Source: CAD feature listing. Evaluate the final solid. Frame: model axes, mm. A direction names the side the tool comes from. Coordinates: 2 decimals unless noted, no trailing zeros. Loops run counter-clockwise (first coordinate to the right, second up) from the corner with the lowest first, then second, coordinate; pieces in that order, holes last.
from build123d import *

# Parameters (mm, degrees)
SKETCH1_W             = 64.8
SKETCH1_H             = 12.6
BOSS_EXTRUDE1_DEPTH   = 2
SKETCH2_W             = 64.8
SKETCH2_H             = 12.6
SKETCH2_W_2           = 60.8
SKETCH2_H_2           = 8.6
BOSS_EXTRUDE2_DEPTH   = 8
CUT_EXTRUDE1_DEPTH    = 67.766758196
BOSS_EXTRUDE3_DEPTH   = 5
BOSS_EXTRUDE3_DRAFT   = 5
BOSS_EXTRUDE3_2_DEPTH = 5
BOSS_EXTRUDE3_2_DRAFT = 5
SKETCH5_R             = 1
CUT_EXTRUDE2_DEPTH    = 4
SKETCH6_W             = 8.6
SKETCH6_H             = 4
CUT_EXTRUDE3_DEPTH    = 3


# Read off the part's stored shape, not the designer's step: Boss-Extrude3
with BuildPart() as part:
    # Sketch1 → Boss-Extrude1 (new body)
    with BuildSketch(Plane(origin=(0, 0, 0), x_dir=(1, 0, 0), z_dir=(0, 1, 0))):
        with Locations((32.4, -6.3)):
            Rectangle(SKETCH1_W, SKETCH1_H)
    extrude(amount=BOSS_EXTRUDE1_DEPTH)

    # Sketch2 → Boss-Extrude2 (add)
    with BuildSketch(Plane(origin=(0, 2, 0), x_dir=(1, 0, 0), z_dir=(0, 1, 0))):
        with Locations((32.4, -6.3)):
            Rectangle(SKETCH2_W, SKETCH2_H)
        with Locations((32.4, -6.3)):
            Rectangle(SKETCH2_W_2, SKETCH2_H_2, mode=Mode.SUBTRACT)
    extrude(amount=BOSS_EXTRUDE2_DEPTH)

    # Sketch3 → Cut-Extrude1 (cut, through all)
    with BuildSketch(Plane(origin=(0, 0, 0), x_dir=(-1, 0, 0), z_dir=(0, -1, 0))):
        with BuildLine():
            ThreePointArc((-24.41, -6.4), (-24.964257247, -4.052128624), (-26.51, -2.2))
            Line((-26.51, -2.2), (-32.81, -2.2))
            ThreePointArc((-32.81, -2.2), (-34.907554575, -6.239778319), (-33.060367627, -10.4))
            Line((-33.060367627, -10.4), (-26.259632373, -10.4))
            ThreePointArc((-26.259632373, -10.4), (-24.894791188, -8.60347112), (-24.41, -6.4))
        make_face()
        with BuildLine():
            ThreePointArc((-33.060367627, -10.4), (-29.66, -11.65), (-26.259632373, -10.4))
            Line((-26.259632373, -10.4), (-33.060367627, -10.4))
        make_face()
        with BuildLine():
            Line((-32.81, -2.2), (-26.51, -2.2))
            ThreePointArc((-26.51, -2.2), (-29.66, -1.15), (-32.81, -2.2))
        make_face()
    extrude(amount=-CUT_EXTRUDE1_DEPTH, mode=Mode.SUBTRACT)


with BuildPart() as boss_extrude3_tool:
    # Boss-Extrude3 outline → Boss-Extrude3 (with draft: the straight prism first)
    with BuildSketch(Plane(origin=(0, 7, 0), x_dir=(1, 0, 0), z_dir=(0, 1, 0))):
        with BuildLine():
            Line((58.936583966, -10.162556682), (61.663416034, -10.162556682))
            ThreePointArc((61.663416034, -10.162556682), (62.076528267, -9.738845855), (62.362556682, -9.220791486))
            Line((62.362556682, -9.220791486), (62.362556682, -7.619208514))
            ThreePointArc((62.362556682, -7.619208514), (61.800640796, -6.794120462), (60.933251192, -6.3))
            ThreePointArc((60.933251192, -6.3), (61.800640796, -5.805879538), (62.362556682, -4.980791486))
            Line((62.362556682, -4.980791486), (62.362556682, -3.379208514))
            ThreePointArc((62.362556682, -3.379208514), (62.076528267, -2.861154145), (61.663416034, -2.437443318))
            Line((61.663416034, -2.437443318), (58.936583966, -2.437443318))
            ThreePointArc((58.936583966, -2.437443318), (58.125947095, -4.590975715), (59.666748808, -6.3))
            ThreePointArc((59.666748808, -6.3), (58.125947095, -8.009024285), (58.936583966, -10.162556682))
        make_face()
    extrude(amount=-BOSS_EXTRUDE3_DEPTH)
    # Boss-Extrude3: the draft: its side faces are tilted about the plane it starts from
    boss_extrude3_sides = [boss_extrude3_tool.faces().sort_by_distance(p)[0] for p in [
        (60.3, 4.5, 10.162556682),
        (62.076528267, 4.5, 9.738845855),
        (62.362556682, 4.5, 8.42),
        (61.800640796, 4.5, 6.794120462),
        (61.800640796, 4.5, 5.805879538),
        (62.362556682, 4.5, 4.18),
        (62.076528267, 4.5, 2.861154145),
        (60.3, 4.5, 2.437443318),
        (58.125947095, 4.5, 4.590975715),
        (58.125947095, 4.5, 8.009024285),
    ]]
    draft(boss_extrude3_sides, Plane(origin=(0, 7, 0), x_dir=(1, 0, 0), z_dir=(0, 1, 0)), BOSS_EXTRUDE3_DRAFT)


with BuildPart() as part_1:
    add(part.part)

    # Boss-Extrude3: add boss_extrude3_tool
    add(boss_extrude3_tool.part)


with BuildPart() as boss_extrude3_2_tool:
    # Boss-Extrude3 2 outline → Boss-Extrude3 2 (with draft: the straight prism first)
    with BuildSketch(Plane(origin=(0, 7, 0), x_dir=(1, 0, 0), z_dir=(0, 1, 0))):
        with BuildLine():
            ThreePointArc((9.64183724, -2), (10.02, -6.392556682), (10.39816276, -2))
            Line((10.39816276, -2), (9.64183724, -2))
        make_face()
    extrude(amount=-BOSS_EXTRUDE3_2_DEPTH)
    # Boss-Extrude3 2: the draft: its side faces are tilted about the plane it starts from
    boss_extrude3_2_sides = [boss_extrude3_2_tool.faces().sort_by_distance(p)[0] for p in [
        (10.02, 4.5, 6.392556682),
        (10.02, 4.5, 2),
    ]]
    draft(boss_extrude3_2_sides, Plane(origin=(0, 7, 0), x_dir=(1, 0, 0), z_dir=(0, 1, 0)), BOSS_EXTRUDE3_2_DRAFT)


with BuildPart() as part_2:
    add(part_1.part)

    # Boss-Extrude3 2: add boss_extrude3_2_tool
    add(boss_extrude3_2_tool.part)

    # Sketch5 → Cut-Extrude2 (cut)
    with BuildSketch(Plane(origin=(0, 7, 0), x_dir=(1, 0, 0), z_dir=(0, 1, 0))):
        with Locations(Location((60.3, -8.42, 0), (0, 0, 270))):
            Circle(SKETCH5_R)
        with Locations(Location((10.02, -4.18, 0), (0, 0, 270))):
            Circle(SKETCH5_R)
        with Locations(Location((60.3, -4.18, 0), (0, 0, 270))):
            Circle(SKETCH5_R)
    extrude(amount=-CUT_EXTRUDE2_DEPTH, mode=Mode.SUBTRACT)

    # Sketch6 → Cut-Extrude3 (cut)
    with BuildSketch(Plane.ZY):
        with Locations((6.3, 5.5)):
            Rectangle(SKETCH6_W, SKETCH6_H)
    extrude(amount=-CUT_EXTRUDE3_DEPTH, mode=Mode.SUBTRACT)


solid = part_2.part
Q1. Section B-B, the plane z = 4.18. Count the separate pieces of the cut face and the enclosed holes in it, plus the area to 3 significant figures.
Q2. Draft query along Z for faces 4 (the flat face through (60, 3, 4)), 5 (the flat face through (64.8, 5, 6)). Return one class per face: +Z half, -Z half, draft (parallel to the pull), parting line (faces both ways), or undercut.
Q3. Section C-C, the plane x = 60.3. Return the cut outline in (y, z), plus the area to 3 significant figures.
Q4. Line query: line 1 along X through (y, z) = (9.5, 5.75); line 2 along Z through (x, y) = (8, 3.25); line 3 along X through (y, z) = (2.5, 7.25). Output: solid intervals per line, ascending.
Q5. Section D-D, the plane z = 8.42. Return the cut outline in (x, y).
Q6. Section A-A, the plane y = 8.75. Return the cut outline in (x, z).
Q7. Access query for faces 1 (the cylindrical face through (59.324, 5.028, 3.963)), 2 (the flat face through (60, 7, 6)), 3 (the flat face through (0, 3, 6)). Directions: +Z, -Z, +X, -X, +Y, -Y. A direction counts if a zero-diameter tool reaches every point of the face in a straight line with its end or side. Return the directions, or none.
Q8. Contact query for flat-ended pins moving along their axis: pin 1 Ø1.6 at (x, z) = (1.5, 6.5) entering from -Y; pin 2 Ø3 at (x, z) = (16.5, 6.5) entering from +Y; pin 3 Ø2 at (x, z) = (9.5, 4) entering from +Y; pin 4 Ø1 at (y, z) = (5.5, 8.5) entering from -X. Output: stop coordinate, or through.
Derived:
1. separate pieces: 3
1. enclosed holes: 0
1. area: 166 mm2
2. face 4: undercut
2. face 5: draft
3. outline: (0, 0) - (10, 0) - (10, 2) - (2, 2) - (7, 2.44) - (7, 3.18) - (3, 3.18) - (3, 5.18) - (7, 5.18) - (7, 7.42) - (3, 7.42) - (3, 9.42) - (7, 9.42) - (7, 10.16) - (2, 10.6) - (10, 10.6) - (10, 12.6) - (0, 12.6) - close
3. area: 82.0 mm2
4. line 1: x = 0 to 2, 62.8 to 64.8
4. line 2: z = 0 to 2, 2.64 to 5.72, 10.6 to 12.6
4. line 3: x = 0 to 2, 57.97 to 62.63, 62.8 to 64.8
5. outline: (0, 0) - (24.81, 0) - (24.81, 2) - (2, 2) - (2, 3.5) - (0, 3.5) - close; (0, 7.5) - (2, 7.5) - (2, 10) - (0, 10) - close; (34.51, 0) - (64.8, 0) - (64.8, 10) - (62.8, 10) - (62.8, 2) - (62.36, 7) - (61.3, 7) - (61.3, 3) - (59.3, 3) - (59.3, 7) - (58.09, 7) - (57.65, 2) - (34.51, 2) - close
6. outline: (0, 0) - (64.8, 0) - (64.8, 12.6) - (0, 12.6) - close; hole (2, 2) - (26.8, 2) arc R5.25 ccw to (32.52, 2) - (62.8, 2) - (62.8, 10.6) - (32.81, 10.6) arc R5.25 ccw to (26.51, 10.6) - (2, 10.6) - close
7. face 1: +Y
7. face 2: -X, +Y
7. face 3: +Z, -Z, -X, +Y, -Y
8. pin 1: stops at y = 0
8. pin 2: stops at y = 2
8. pin 3: stops at y = 7
8. pin 4: stops at x = 57.91
